```python
from build123d import *

# Parameters (mm, degrees)
SKETCH2_W           = 25.4
SKETCH2_H           = 25.4
BOSS_EXTRUDE1_DEPTH = 41.275
SKETCH3_R           = 6.35
SKETCH3_W           = 28.575
SKETCH3_H           = 6.35
SKETCH3_W_2         = 25.4
SKETCH3_H_2         = 9.525
CUT_EXTRUDE1_DEPTH  = 51.100654936
SKETCH4_R           = 3.175
CUT_EXTRUDE2_DEPTH  = 51.100654936


with BuildPart() as part:
    # Sketch2 → Boss-Extrude1 (new, symmetric)
    with BuildSketch(Plane.XY):
        Rectangle(SKETCH2_W, SKETCH2_H)
    extrude(amount=BOSS_EXTRUDE1_DEPTH, both=True)

    # Sketch3 → Cut-Extrude1 (cut, through all)
    with BuildSketch(Plane(origin=(12.7, 0, 0), x_dir=(0, 0, -1), z_dir=(1, 0, 0))):
        Circle(SKETCH3_R)
        with Locations((-26.9875, 9.525)):
            Rectangle(SKETCH3_W, SKETCH3_H)
        with Locations((-26.9875, -9.525)):
            Rectangle(SKETCH3_W, SKETCH3_H)
        with Locations((28.575, 0)):
            Rectangle(SKETCH3_W_2, SKETCH3_H_2)
    extrude(amount=-CUT_EXTRUDE1_DEPTH, mode=Mode.SUBTRACT)

    # Sketch4 → Cut-Extrude2 (cut, through all)
    with BuildSketch(Plane(origin=(0, 12.7, 0), x_dir=(1, 0, 0), z_dir=(0, 1, 0))):
        with Locations(Location((0, 28.575, 0), (0, 0, 270))):
            Circle(SKETCH4_R)
        with Locations(Location((0, -28.575, 0), (0, 0, 270))):
            Circle(SKETCH4_R)
        with BuildLine():
            Line((-12.7, 28.575), (-12.7, 47.625))
            Line((-12.7, 47.625), (12.7, 47.625))
            Line((12.7, 47.625), (12.7, 28.575))
            ThreePointArc((12.7, 28.575), (0, 41.275), (-12.7, 28.575))
        make_face()
        with BuildLine():
            Line((-12.7, -28.575), (-12.7, -47.625))
            Line((-12.7, -47.625), (12.7, -47.625))
            Line((12.7, -47.625), (12.7, -28.575))
            ThreePointArc((12.7, -28.575), (0, -41.275), (-12.7, -28.575))
        make_face()
    extrude(amount=-CUT_EXTRUDE2_DEPTH, mode=Mode.SUBTRACT)


solid = part.part
```
Input: part model. Units: mm. Frame: model coordinates. A direction names the side the tool comes from. Give positions to 0.01 mm unless a question says otherwise; leave off trailing zeros. Loops run counter-clockwise (first coordinate to the right, second up) from the corner with the lowest first, then second, coordinate; pieces in that order, holes last.
1) Section query A-A on y = 0. Return the cut outline in (x, z) (3 decimals).
A:
outline: (-12.7, -15.875) - (12.7, -15.875) - (12.7, -6.35) - (-12.7, -6.35) - close; (-12.7, 6.35) - (12.7, 6.35) - (12.7, 28.575) arc R12.7 ccw to (-12.7, 28.575) - close; hole circle Ø6.35 at (0, 28.575)
2) Line query: L1, parallel to Y at x = 9.5, z = -32; L2, parallel to Z at x = -0.25, y = -0.5 (3 decimals); L3, parallel to Z at x = 5.5, y = 4.25 (3 decimals). Output: solid intervals per line, ascending.
A:
L1: y = -12.7 to -4.76, 4.76 to 12.7
L2: z = -15.875 to -6.33, 6.33 to 25.41, 31.74 to 41.273
L3: z = -15.875 to -4.718, 4.718 to 40.022
3) Reachability of faces 1 (the flat face through (0, 6.35, 24)), 2 (the flat face through (-3, 4.762, -26)), 3 (the flat face through (0, -6.35, 24)) from +Z, -Z, +X, -X, +Y, -Y: full face, straight path, thin tool, end or side. Return the list, or none.
A:
face 1: +Z, +X, -X, +Y
face 2: -Z, +X, -X
face 3: +Z, +X, -X, -Y
4) Section query B-B on x = 0. Count the separate pieces of the cut face and the enclosed holes in it, and give its area (3 significant figures).
A:
separate pieces: 4
enclosed holes: 1
area: 1,180 mm2
5) Contact query for flat-ended pins moving along their axis: pin 1 (7.5 mm diameter, centred on x = -4, z = 24.5, fed in from +Y); pin 2 (3 mm diameter, centred on x = -7.5, y = 5, fed in from +Z); pin 3 (10 mm diameter, centred on y = 0, z = 0, fed in from +X); pin 4 (3 mm diameter, centred on x = -0.5, y = 8.5, fed in from +Z). Output: stop coordinate, or through.
A:
pin 1: stops at y = 6.35
pin 2: stops at z = 39.77
pin 3: passes through
pin 4: stops at z = 12.7
6) Mould query, pull axis Z, two halves, no side actions, for faces 4 (the cylindrical face through (-1.932, 0.089, 26.055)), 5 (the flat face through (12.7, 3, -6)), 6 (the flat face through (0, -10, 12.7)). Classes: released by +Z, released by -Z, zero draft, split by the parting line, or undercut.
A:
face 4: undercut
face 5: zero draft
face 6: released by +Z
7) Section query C-C on z = 0. Return the cut outline in (x, y).
A:
outline: (-12.7, -12.7) - (12.7, -12.7) - (12.7, -6.35) - (-12.7, -6.35) - close; (-12.7, 6.35) - (12.7, 6.35) - (12.7, 12.7) - (-12.7, 12.7) - close
8) Section query D-D on y = 7.75. Return the cut outline in (x, z) (3 decimals), and give its area (3 significant figures).
A:
outline: (-12.7, -28.575) arc R12.7 ccw to (12.7, -28.575) - (12.7, 12.7) - (-12.7, 12.7) - close; hole circle Ø6.35 at (0, -28.575)
area: 1,270 mm2
